Work out the finished part from the listing and answer in its coordinate system (mm). A direction names the side the tool comes from. Coordinates: 2 decimals unless noted, no trailing zeros. Loops run counter-clockwise (first coordinate to the right, second up) from the corner with the lowest first, then second, coordinate; pieces in that order, holes last. Notation, with made-up numbers: (-34.75, -9.75) - (5.25, -9.75) arc R19 cw to (5.25, 24.25) - close; hole circle Ø5 at (4.5, 26). An arc over 180 degrees is marked (long way). Write each question's results on one line, items separated by ' | '. Start each with the question number.
Item 1: For a pull along X with two mould halves and no side action, classify faces 3 (the face through (61.5, 20.51, 25.85)), 4 (the face through (51.58, 20.51, 42.24)), 5 (the face through (24, 20.6, 0)) as +X half, -X half, draft (parallel to the pull), parting line (faces both ways), or undercut.
Item 2: Section D-D, the plane x = 5 is taken. Write down the section's boundary in (y, z).
Item 3: Each of these flat-tipped pins is pushed along its axis until it touches: pin 1 Ø3 at (y, z) = (13.5, 42.5) entering from +X; pin 2 Ø1 at (y, z) = (3, 42.5) entering from -X; pin 3 Ø1.9 at (x, z) = (53, 10.5) entering from -Y; pin 4 Ø2 at (x, z) = (41.5, 37) entering from -Y. Where does it stop, or does it pass through?
Item 4: Section C-C, the plane z = 41.5 is taken. Count the separate pieces of the cut face and the enclosed holes in it, plus the area to 3 significant figures.
Item 5: Consider probe 1 along Z at (x, y) = (84, 20.4); probe 2 along Y at (x, z) = (16, 16.5); probe 3 along X at (y, z) = (16.5, 5). Determine where each line is inside the solid, lowest interval first. Write a range as [from, to].
Item 6: Section A-A, the plane x = 53 is taken. Write down the section's boundary in (y, z), plus the area to 3 significant figures.
Item 7: Section B-B, the plane x = 78 is taken. Write down the section's boundary in (y, z).
Item 8: A tool of negligible diameter and unlimited length cuts with its end or side. For faces 1 (the face through (46, 20, 26)), 2 (the face through (44, 21, 26)), from which of +Z, -Z, +X, -X, +Y, -Y can it reach the whole face along a straight path? Write none if from no direction.
from build123d import *

# Parameters (mm, degrees)
EXTRUDE_1_DEPTH     = 52
SKETCH_3_R          = 1.6
CUT_EXTRUDE_1_DEPTH = 52


with BuildPart() as part:
    # 草图2 → 凸台-拉伸1 (new body)
    with BuildSketch(Plane.XY):
        with BuildLine():
            Line((0, 21), (90, 21))
            Line((90, 21), (90, 20))
            Line((90, 20), (0, 20))
            add(Edge.make_bspline(
                [(0, 20), (-11.918826451, 20), (-19.365080243, 9.425379896), (-23.265119014, 0)],
                knots=[0, 0, 0, 0, 1, 1, 1, 1], degree=3))
            Line((-23.265119014, 0), (-23.265119014, -1.344088089))
            Line((-23.265119014, -1.344088089), (-25.409868427, -1.344088089))
            Line((-25.409868427, -1.344088089), (-25.409868427, 0))
            add(Edge.make_bspline(
                [(0, 21), (-12.514575739, 21), (-20.585292942, 9.393477036), (-25.409868427, 0)],
                knots=[0, 0, 0, 0, 1, 1, 1, 1], degree=3))
        make_face()
    extrude(amount=EXTRUDE_1_DEPTH)

    # 草图3 → 切除-拉伸1 (cut)
    with BuildSketch(Plane(origin=(0, 21, 0), x_dir=(1, 0, 0), z_dir=(0, 1, 0))):
        with Locations(Location((84, -10.5, 0), (0, 0, 270))):
            Circle(SKETCH_3_R)
        with Locations(Location((84, -41.5, 0), (0, 0, 270))):
            Circle(SKETCH_3_R)
        with Locations(Location((53, -41.5, 0), (0, 0, 270))):
            Circle(SKETCH_3_R)
        with Locations(Location((53, -10.5, 0), (0, 0, 270))):
            Circle(SKETCH_3_R)
        with BuildLine():
            Line((90, -19), (68.5, -19))
            ThreePointArc((68.5, -19), (61.5, -26), (68.5, -33))
            Line((68.5, -33), (90, -33))
            Line((90, -33), (90, -19))
        make_face()
    extrude(amount=-CUT_EXTRUDE_1_DEPTH, mode=Mode.SUBTRACT)


solid = part.part
Answer key:
1) face 3: +X half | face 4: undercut | face 5: draft
2) outline: (20, 0) - (21, 0) - (21, 52) - (20, 52) - close
3) pin 1: stops at x = -13.05 | pin 2: stops at x = -24.07 | pin 3: passes through | pin 4: stops at y = 20
4) separate pieces: 3 | enclosed holes: 0 | area: 126 mm^2
5) probe 1: z = [0, 8.9], [12.1, 19], [33, 39.9], [43.1, 52] | probe 2: y = [20, 21] | probe 3: x = [-12.72, -11.08]
6) outline: (20, 0) - (21, 0) - (21, 8.9) - (20, 8.9) - close; (20, 12.1) - (21, 12.1) - (21, 39.9) - (20, 39.9) - close; (20, 43.1) - (21, 43.1) - (21, 52) - (20, 52) - close | area: 45.6 mm^2
7) outline: (20, 0) - (21, 0) - (21, 19) - (20, 19) - close; (20, 33) - (21, 33) - (21, 52) - (20, 52) - close
8) face 1: +Z, -Z, +X, -Y | face 2: +Z, -Z, +X, -X, +Y
